```python
from build123d import *

# Parameters (mm, degrees)
SKETCH1_W                  = 101.5
SKETCH1_H                  = 114.5
TR_KKPLAAT_DEPTH           = 1.5
SKETCH2_R                  = 1.5
AUGUD_DEPTH                = 1.5
SKETCH3_W                  = 35.5
SKETCH3_H                  = 13
EXP_CONN_A_B_DEPTH         = 2.5
SKETCH4_W                  = 13
SKETCH4_H                  = 8
LCD_CONN_A_B_DEPTH         = 2.5
SKETCH5_W                  = 13
SKETCH5_H                  = 5
WIFI_BT_DEPTH              = 2.5
SKETCH6_W                  = 17
SKETCH6_H                  = 5
JTAG_DEPTH                 = 5
SKETCH7_W                  = 9
SKETCH7_H                  = 15
HDMI_A_B_DEPTH             = 6
SKETCH8_W                  = 25.5
SKETCH8_H                  = 16
USB_ETHERNET_DEPTH         = 29
SKETCH9_W                  = 14
SKETCH9_H                  = 9
F_5V_IN_DEPTH              = 10
SKETCH10_W                 = 12
SKETCH10_H                 = 12
HEADPHONE_DEPTH            = 24.5
SKETCH11_W                 = 8
SKETCH11_H                 = 8
MINI_USB_DEPTH             = 4
SKETCH12_W                 = 30
SKETCH12_H                 = 4
BOSS_EXTRUDE11_DEPTH       = 10.5
BOSS_EXTRUDE12_DEPTH       = 5
SKETCH14_W                 = 18
SKETCH14_H                 = 27
SD_CARD_SLOT_DEPTH         = 3
SKETCH15_W                 = 1.5
SKETCH15_H                 = 3
STATUS_LED_DEPTH           = 0.5
SKETCH16_W                 = 6
SKETCH16_H                 = 6
PWRON_RESET_GPIO_121_DEPTH = 4
SKETCH17_W                 = 20
SKETCH17_H                 = 6.5
CAMERA_CONN_DEPTH          = 1
SKETCH18_R                 = 1
WIFI_BT_ANTENNA_DEPTH      = 3


with BuildPart() as part:
    # Sketch1 → trükkplaat (new body)
    with BuildSketch(Plane(origin=(0, 0, 0), x_dir=(1, 0, 0), z_dir=(0, 1, 0))):
        Rectangle(SKETCH1_W, SKETCH1_H)
    extrude(amount=TR_KKPLAAT_DEPTH)

    # Sketch2 → augud (cut)
    with BuildSketch(Plane(origin=(0, 1.5, 0), x_dir=(1, 0, 0), z_dir=(0, 1, 0))):
        with Locations(Location((-47, 53.5, 0), (0, 0, 270))):
            Circle(SKETCH2_R)
        with Locations(Location((47, 53.5, 0), (0, 0, 270))):
            Circle(SKETCH2_R)
        with Locations(Location((47, -53.5, 0), (0, 0, 270))):
            Circle(SKETCH2_R)
        with Locations(Location((-47, -53.5, 0), (0, 0, 270))):
            Circle(SKETCH2_R)
        with Locations(Location((-21, 53.5, 0), (0, 0, 270))):
            Circle(SKETCH2_R)
        with Locations(Location((-21, -16.5, 0), (0, 0, 270))):
            Circle(SKETCH2_R)
        with Locations(Location((47, -16.5, 0), (0, 0, 270))):
            Circle(SKETCH2_R)
    extrude(amount=-AUGUD_DEPTH, mode=Mode.SUBTRACT)

    # Sketch3 → exp. conn. A/B (add)
    with BuildSketch(Plane(origin=(0, 1.5, 0), x_dir=(1, 0, 0), z_dir=(0, 1, 0))):
        with Locations((2, 47.75)):
            Rectangle(SKETCH3_W, SKETCH3_H)
    extrude(amount=EXP_CONN_A_B_DEPTH)

    # Sketch4 → LCD conn. A/B (add)
    with BuildSketch(Plane(origin=(0, 1.5, 0), x_dir=(1, 0, 0), z_dir=(0, 1, 0))):
        with Locations((29.25, 51.25)):
            Rectangle(SKETCH4_W, SKETCH4_H)
    extrude(amount=LCD_CONN_A_B_DEPTH)

    # Sketch5 → WIFI/BT (add)
    with BuildSketch(Plane(origin=(0, 1.5, 0), x_dir=(1, 0, 0), z_dir=(0, 1, 0))):
        with Locations((-32.75, 51.75)):
            Rectangle(SKETCH5_W, SKETCH5_H)
    extrude(amount=WIFI_BT_DEPTH)

    # Sketch6 → JTAG (add)
    with BuildSketch(Plane(origin=(0, 1.5, 0), x_dir=(1, 0, 0), z_dir=(0, 1, 0))):
        with Locations((7.25, 31.75)):
            Rectangle(SKETCH6_W, SKETCH6_H)
    extrude(amount=JTAG_DEPTH)

    # Sketch7 → HDMI A/B (add)
    with BuildSketch(Plane(origin=(0, 1.5, 0), x_dir=(1, 0, 0), z_dir=(0, 1, 0))):
        with Locations((47.25, 40.75)):
            Rectangle(SKETCH7_W, SKETCH7_H)
        with Locations((48.068861521, 17.75)):
            Rectangle(SKETCH7_W, SKETCH7_H)
    extrude(amount=HDMI_A_B_DEPTH)

    # Sketch8 → USB/Ethernet (add)
    with BuildSketch(Plane(origin=(0, 1.5, 0), x_dir=(1, 0, 0), z_dir=(0, 1, 0))):
        with Locations((38, -3.75)):
            Rectangle(SKETCH8_W, SKETCH8_H)
    extrude(amount=USB_ETHERNET_DEPTH)

    # Sketch9 → 5V in (add)
    with BuildSketch(Plane(origin=(0, 1.5, 0), x_dir=(1, 0, 0), z_dir=(0, 1, 0))):
        with Locations((43.75, -25.25)):
            Rectangle(SKETCH9_W, SKETCH9_H)
    extrude(amount=F_5V_IN_DEPTH)

    # Sketch10 → Headphone (add)
    with BuildSketch(Plane(origin=(0, 1.5, 0), x_dir=(1, 0, 0), z_dir=(0, 1, 0))):
        with Locations((44.75, -40.75)):
            Rectangle(SKETCH10_W, SKETCH10_H)
    extrude(amount=HEADPHONE_DEPTH)

    # Sketch11 → mini-USB (add)
    with BuildSketch(Plane(origin=(0, 1.5, 0), x_dir=(1, 0, 0), z_dir=(0, 1, 0))):
        with Locations((25.75, -55.25)):
            Rectangle(SKETCH11_W, SKETCH11_H)
    extrude(amount=MINI_USB_DEPTH)

    # Sketch12 → Boss-Extrude11 (add)
    with BuildSketch(Plane(origin=(0, 1.5, 0), x_dir=(1, 0, 0), z_dir=(0, 1, 0))):
        with Locations((-28.25, -55.25)):
            Rectangle(SKETCH12_W, SKETCH12_H)
    extrude(amount=BOSS_EXTRUDE11_DEPTH)

    # Sketch13 → Boss-Extrude12 (add)
    with BuildSketch(Plane.XY.offset(57.25)):
        with BuildLine():
            Line((-36.25, 10.75), (-20.25, 10.75))
            ThreePointArc((-20.25, 10.75), (-16.25, 6.75), (-20.25, 2.75))
            Line((-20.25, 2.75), (-36.25, 2.75))
            ThreePointArc((-36.25, 2.75), (-40.25, 6.75), (-36.25, 10.75))
        make_face()
    extrude(amount=BOSS_EXTRUDE12_DEPTH)

    # Sketch14 → SD-card slot (add)
    with BuildSketch(Plane(origin=(0, 1.5, 0), x_dir=(1, 0, 0), z_dir=(0, 1, 0))):
        with Locations((-41.75, -27.75)):
            Rectangle(SKETCH14_W, SKETCH14_H)
    extrude(amount=SD_CARD_SLOT_DEPTH)

    # Sketch15 → status LED (add)
    with BuildSketch(Plane(origin=(0, 1.5, 0), x_dir=(1, 0, 0), z_dir=(0, 1, 0))):
        with Locations((-48, -4.75)):
            Rectangle(SKETCH15_W, SKETCH15_H)
        with Locations((-48, 5.25)):
            Rectangle(SKETCH15_W, SKETCH15_H)
    extrude(amount=STATUS_LED_DEPTH)

    # Sketch16 → PWRON_RESET/GPIO_121 (add)
    with BuildSketch(Plane(origin=(0, 1.5, 0), x_dir=(1, 0, 0), z_dir=(0, 1, 0))):
        with Locations((-5.75, -33.25)):
            Rectangle(SKETCH16_W, SKETCH16_H)
        with Locations((-17.25, -33.25)):
            Rectangle(SKETCH16_W, SKETCH16_H)
    extrude(amount=PWRON_RESET_GPIO_121_DEPTH)

    # Sketch17 → camera conn (add)
    with BuildSketch(Plane(origin=(0, 1.5, 0), x_dir=(1, 0, 0), z_dir=(0, 1, 0))):
        with Locations((4.75, -54)):
            Rectangle(SKETCH17_W, SKETCH17_H)
    extrude(amount=CAMERA_CONN_DEPTH)

    # Sketch18 → WIFI?/BT? antenna (add)
    with BuildSketch(Plane(origin=(0, 1.5, 0), x_dir=(1, 0, 0), z_dir=(0, 1, 0))):
        with Locations(Location((-32.75, 31.25, 0), (0, 0, 90))):
            Circle(SKETCH18_R)
    extrude(amount=WIFI_BT_ANTENNA_DEPTH)


solid = part.part
```
Could you check a few things on this model? Use its own coordinates, in mm. A direction names the side the tool comes from. Coordinates: 2 decimals unless noted, no trailing zeros. Loops run counter-clockwise (first coordinate to the right, second up) from the corner with the lowest first, then second, coordinate; pieces in that order, holes last. Notation, with made-up numbers: M 17,-10.75 L 48,-10.75 A28 cw 48,20.25 Z; hole C 43,8 d8. An arc over 180 degrees is marked long. Put each result on its own line as item: value. Start each with the question number.
(1) Suppose I cut it at D-D on z = -38. Please give me the cut outline in (x, y), then the cut area to 3 significant figures.
(2) I need wall thicknesses on line 1 (X direction, y = 0.9, z = 53.5); line 2 (X direction, y = 0.6, z = -53.5); line 3 (X direction, y = 1.1, z = 16.5). Which ranges of each line are inside material? Lowest first, please. Write a range as from..to.
(3) For faces 1 (the face through (-26.25, 3, -52)), 2 (the face through (-16.25, 6.84, 59.72)), 3 (the face through (-42, 3, 41.25)), 4 (the face through (-2.75, 3, 33)), 5 (the face through (-17, 3, 30.25)), which set-ups out of +Z, -Z, +X, -X, +Y, -Y let a thin tool reach every point of the face, with its end or its side?
(4) Thinking about a two-plate mould opening in Z: for faces 6 (the face through (-39.25, 3, -52)), 7 (the face through (29, 3, -47.25)), 8 (the face through (-15, 4, 57.25)), which applies, pulls with the +Z half, pulls with the -Z half, needs draft (parallel to the pull), parting line crosses it, or undercut?
(5) Will these pins go through, and if not, where does the flat tip stop? P1, Ø0.8, axis at y = 3.5, z = -52, coming from the +X side; P2, Ø2, axis at x = -26, z = 55, coming from the +Y side; P3, Ø3, axis at x = -9, y = 5.5, coming from the +Z side.
(6) Suppose I cut it at C-C on x = 47. Count the separate pieces of the cut face and the enclosed holes in it, then the cut area to 3 significant figures.
(7) Suppose I cut it at A-A on y = 18.5. Please give me the cut outline in (x, z).
(8) Suppose I cut it at B-B on z = 22.5. Please give me the cut outline in (x, y).
Solutions:
1. outline: M -50.75,0 L 50.75,0 L 50.75,1.5 L 51.75,1.5 L 51.75,7.5 L 42.75,7.5 L 42.75,1.5 L -50.75,1.5 Z
1. area: 206 mm2
2. line 1: x = -50.75..-48.5, -45.5..45.5, 48.5..50.75
2. line 2: x = -50.75..-48.5, -45.5..-22.5, -19.5..45.5, 48.5..50.75
2. line 3: x = -50.75..-22.5, -19.5..45.5, 48.5..50.75
3. face 1: -Z, +Y
3. face 2: +Z
3. face 3: -X, +Y
3. face 4: +Y
3. face 5: +X, +Y
4. face 6: needs draft
4. face 7: undercut
4. face 8: pulls with the +Z half
5. P1: stops at x = 35.75
5. P2: stops at y = 12
5. P3: stops at z = 36.25
6. separate pieces: 4
6. enclosed holes: 0
6. area: 1,190 mm2
7. outline: M 25.25,-4.25 L 50.75,-4.25 L 50.75,11.75 L 25.25,11.75 Z; M 38.75,34.75 L 50.75,34.75 L 50.75,46.75 L 38.75,46.75 Z
8. outline: M -50.75,0 L 50.75,0 L 50.75,11.5 L 36.75,11.5 L 36.75,1.5 L -32.75,1.5 L -32.75,4.5 L -50.75,4.5 Z
